Part model, mm, in its own coordinate system. A direction names the side the tool comes from. Round coordinates to 2 decimals unless told otherwise and drop trailing zeros. Order: outer loops, then holes, each group sorted by start corner. A loop starts at its lowest first (then second) coordinate and runs counter-clockwise, first axis right, second up. Notation, with made-up numbers: M 47.25,81.5 L 68.25,81.5 A24 cw 68.25,118.5 Z; hole C 9.5,52.5 d3. An arc over 180 degrees is marked long. Write each question's results on one line, items separated by ' | '. Start each with the question number.
1. Band-saw the part on C-C, the plane x = -61. List the corners of the cut face in (y, z).
2. Two-plate mould, pull along X, no slides. Class faces 4 (the face through (-2, 0, 0)), 5 (the face through (173, 0, 31)), 6 (the face through (-2, 0, 2)), 7 (the face through (161, -3, 25)): +X half, -X half, draft (parallel to the pull), parting line (faces both ways), or undercut.
3. Band-saw the part on B-B, the plane y = 0. List the corners of the cut face in (x, z), then the cut area to 3 significant figures.
4. Band-saw the part on A-A, the plane z = 41. List the corners of the cut face in (x, y), then the cut area to 3 significant figures.
5. Which spindle directions (+Z, -Z, +X, -X, +Y, -Y) get a long thin tool onto all of the face, cutting with end or side? Do faces 1 (the face through (163, -3, 21)), 2 (the face through (-173, 0, 31)), 3 (the face through (-161, 3, 25)). Say none if no direction does.
6. Drop flat-ended pins along their axis: pin 1 Ø4 at (x, y) = (168, -1.5) entering from +Z; pin 2 Ø2 at (x, y) = (-168.5, 4.5) entering from +Z. Give the stop position or say it passes through.
7. Probe L1, parallel to X at y = -2.25, z = 24; L2, parallel to X at y = -5.5, z = 5; L3, parallel to X at y = 2.5, z = 58.5. List the from-to ranges inside material, lowest first. Write a range as [from, to].
Autodesk Fusion 360 part; units mm, degrees
sketch "Sketch1" plane through (0, 0, 0) normal (0, 0, 1) x (1, 0, 0)
  line L0 (-173, 6) -> (173, 6)
  line L1 (173, 6) -> (173, -6)
  line L2 (173, -6) -> (-173, -6)
  line L3 (-173, -6) -> (-173, 6)
  dimension "d1" = 346
  dimension "d2" = 12
extrude "Extrude1" add sketch "Sketch1" along normal blind 2
sketch "Sketch2" plane through (0, 0, 2) normal (0, 0, 1) x (-1, 0, 0)
  line L0 (173, 6) -> (-173, 6)
  line L1 (-173, 6) -> (-173, -6)
  line L2 (-173, -6) -> (173, -6)
  line L3 (173, -6) -> (173, 6)
  line L4 (-171, 6) -> (-171, -6)
  line L5 (-171, 6) -> (-173, 6)
  line L6 (-173, -6) -> (-171, -6)
  line L7 (171, 6) -> (171, -6)
  line L8 (171, 6) -> (173, 6)
  line L9 (173, -6) -> (171, -6)
  dimension "d9" = 2
  dimension "d10" = 2
extrude "Extrude2" add sketch "Sketch2" along normal blind 60 contours L0 L2 L3 L7 L8 L9 | L0 L1 L2 L4 L5 L6
sketch "Sketch3" plane through (171, 0, 0) normal (-1, 0, 0) x (0, -1, 0)
  line L0 (-6, 2) -> (6, 2)
  line L1 (6, 2) -> (6, 62)
  line L2 (6, 62) -> (-6, 62)
  line L3 (-6, 62) -> (-6, 2)
  line L4 (-6, 62) -> (-6, 47)
  line L5 (-6, 47) -> (6, 47)
  line L6 (6, 47) -> (6, 0)
  line L7 (6, 0) -> (-6, 0)
  line L8 (-6, 0) -> (-6, 47)
  dimension "d13" = 15
extrude "Extrude3" add sketch "Sketch3" along normal blind 10 contours L0 L1 L3 L5 L6 L8
sketch "Sketch4" plane through (0, 0, 47) normal (0, 0, 1) x (-1, 0, 0)
  line L0 (-171, 6) -> (-171, -6)
  line L1 (-171, -6) -> (-161, -6)
  line L2 (-161, -6) -> (-161, 6)
  line L3 (-161, 6) -> (-171, 6)
  line L4 (-171, 4.5) -> (-170, 4.5)
  line L5 (-170, 4.5) -> (-163, 4.5)
  line L6 (-163, 4.5) -> (-163, -4.5)
  line L7 (-163, -4.5) -> (-171, -4.5)
  line L8 (-171, 4.5) -> (-171, 3.6158)
  dimension "d16" = 1.5
  dimension "d17" = 1.5
  dimension "d18" = 8
extrude "Extrude4" cut sketch "Sketch4" against normal blind 43 contours L0 L4 L5 L6 L7 L8
sketch "Sketch5" plane through (161, 0, 0) normal (-1, 0, 0) x (0, -1, 0)
  line L0 (-6, 47) -> (-6, 2)
  line L1 (-6, 2) -> (6, 2)
  line L2 (6, 2) -> (6, 47)
  line L3 (6, 47) -> (-6, 47)
  line L4 (-6, 47) -> (6, 47)
  line L5 (0, 47) -> (-2, 47)
  line L6 (3, 12) -> (3, 13.1676)
  line L7 (-2, 47) -> (-2, 14)
  line L8 (2, 14) -> (2, 47)
  line L9 (2, 47) -> (-2, 47)
  arc A0 (0, 12) -> (2, 14) centre (0, 14) ccw
  arc A1 (-2, 14) -> (0, 12) centre (0, 14) ccw
  point P0 (-2, 12)
  point P1 (3.9688, 12.6113)
  point P2 (-2, 12)
  point P3 (2, 12)
  dimension "d21" = 2
  dimension "d30" = 35
  dimension "d31" = 4
  dimension "d32" = 35
  dimension "d33" = 2
  dimension "d34" = 2
extrude "Extrude5" cut sketch "Sketch5" against normal blind 2 contours L3 L4 L5 L7 L8 L9 A0 A1
sketch "Sketch6" plane through (-171, 0, 0) normal (1, 0, 0) x (0, 1, 0)
  line L0 (-6, 2) -> (6, 2)
  line L1 (6, 2) -> (6, 62)
  line L2 (6, 62) -> (-6, 62)
  line L3 (-6, 62) -> (-6, 2)
  line L4 (-6, 62) -> (-6, 47)
  line L5 (-6, 47) -> (6, 47)
  line L6 (-6, 47) -> (-6, 0)
  line L7 (-6, 0) -> (6, 0)
  line L8 (6, 0) -> (6, 47)
  dimension "d37" = 15
extrude "Extrude6" add sketch "Sketch6" along normal blind 10 contours L0 L1 L3 L5 L6 L8
sketch "Sketch7" plane through (0, 0, 47) normal (0, 0, 1) x (-1, 0, 0)
  line L0 (171, -6) -> (171, 6)
  line L1 (171, 6) -> (161, 6)
  line L2 (161, 6) -> (161, -6)
  line L3 (161, -6) -> (171, -6)
  line L4 (171, 4.5) -> (163, 4.5)
  line L5 (163, 4.5) -> (163, -4.5)
  line L6 (163, -4.5) -> (171, -4.5)
  dimension "d40" = 1.5
  dimension "d41" = 1.5
  dimension "d42" = 2
extrude "Extrude7" cut sketch "Sketch7" against normal blind 43 contours L0 L4 L5 L6
sketch "Sketch8" plane through (-161, 0, 0) normal (1, 0, 0) x (0, 1, 0)
  line L0 (-6, 47) -> (-6, 2)
  line L1 (-6, 2) -> (6, 2)
  line L2 (6, 2) -> (6, 47)
  line L3 (6, 47) -> (-6, 47)
  line L4 (6, 47) -> (-6, 47)
  line L5 (0, 47) -> (-2, 47)
  line L6 (-2, 47) -> (-2, 14)
  line L7 (2, 14) -> (2, 47)
  line L8 (2, 47) -> (-2, 47)
  arc A0 (-2, 14) -> (0, 12) centre (0, 14) ccw
  arc A1 (0, 12) -> (2, 14) centre (0, 14) ccw
  point P0 (-2, 12)
  point P1 (2, 12)
  dimension "d45" = 2
  dimension "d46" = 35
  dimension "d47" = 4
  dimension "d48" = 35
  dimension "d49" = 2
  dimension "d50" = 2
extrude "Extrude8" cut sketch "Sketch8" against normal blind 2 contours L3 L4 L5 L6 L7 L8 A0 A1
Solution:
1) outline: M -6,0 L 6,0 L 6,2 L -6,2 Z
2) face 4: draft | face 5: +X half | face 6: undercut | face 7: undercut
3) outline: M -173,0 L 173,0 L 173,62 L 171,62 L 171,4 L 163,4 L 163,12 L 161,12 L 161,2 L -161,2 L -161,12 L -163,12 L -163,4 L -171,4 L -171,62 L -173,62 Z | area: 1,000 mm^2
4) outline: M -173,-6 L -161,-6 L -161,-2 L -163,-2 L -163,-4.5 L -171,-4.5 L -171,4.5 L -163,4.5 L -163,2 L -161,2 L -161,6 L -173,6 Z; M 161,-6 L 173,-6 L 173,6 L 161,6 L 161,2 L 163,2 L 163,4.5 L 171,4.5 L 171,-4.5 L 163,-4.5 L 163,-2 L 161,-2 Z | area: 128 mm^2
5) face 1: +Z | face 2: +Z, -Z, -X, +Y, -Y | face 3: +Z, +Y, -Y
6) pin 1: z = 4 | pin 2: z = 47
7) L1: [-173, -171], [-163, -161], [161, 163], [171, 173] | L2: [-173, -161], [161, 173] | L3: [-173, -171], [171, 173]
